```python
from build123d import *

# Parameters (mm, degrees)
F0_W      = 85
F0_H      = 117
F1_DEPTH  = 4
F2_W      = 2
F2_H      = 5
F3_DEPTH  = 7
F4_W      = 2
F4_H      = 4.0044696238
F5_DEPTH  = 5
F6_R      = 1
F7_R      = 1
F8_R      = 2
F11_W     = 117
F11_H     = 4
F12_DEPTH = 3
F10_W     = 117
F10_H     = 4
F14_DEPTH = 3
F13_W     = 85
F13_H     = 3
F13_W_2   = 3
F13_H_2   = 117
F15_DEPTH = 25
F16_DEPTH = 3
F18_DEPTH = 3
F19_R     = 0.75
F20_DEPTH = 4
F21_DEPTH = 3
F23_DEPTH = 3


# Not quite as in the source:
# - a feature names something its author has since deleted; it is built from what else it names


with BuildPart() as f1:
    # F0 (on Top) → F1 (new body)
    with BuildSketch(Plane.XY):
        Rectangle(F0_W, F0_H)
    extrude(amount=F1_DEPTH)

    # F2 (on face) → F3 (join)
    with BuildSketch(Plane(origin=(0, 0, 0), x_dir=(1, 0, 0), z_dir=(0, 0, -1))):
        with Locations((-21, -36)):
            Rectangle(F2_W, F2_H)
    extrude(amount=F3_DEPTH)

    # F4 (on face) → F5 (join)
    with BuildSketch(Plane(origin=(0, 38.5, 0), x_dir=(-1, 0, 0), z_dir=(0, 1, 0))):
        with Locations((21, -4.9977651881)):
            Rectangle(F4_W, F4_H)
    extrude(amount=F5_DEPTH)

    # F6
    f6_edges = [f1.edges().sort_by_distance(p)[0] for p in [
        (-21, 43.5, -2.99553),
    ]]
    fillet(f6_edges, radius=F6_R)

    # F7
    f7_edges = [f1.edges().sort_by_distance(p)[0] for p in [
        (-21, 43.5, -7),
    ]]
    fillet(f7_edges, radius=F7_R)

    # F8
    f8_edges = [f1.edges().sort_by_distance(p)[0] for p in [
        (-21, 33.5, -7),
    ]]
    fillet(f8_edges, radius=F8_R)


with BuildPart() as f9_1:
    # F9: instance of F1
    add(f1.part.mirror(Plane.YZ))


with BuildPart() as f1_1:
    add(f1.part)

    add(f9_1.part)  # F12 merges F9_1
    # F11 (on face) → F12 (join)
    with BuildSketch(Plane(origin=(-42.5, 0, 0), x_dir=(0, -1, 0), z_dir=(-1, 0, 0))):
        with Locations((0, 2)):
            Rectangle(F11_W, F11_H)
    extrude(amount=F12_DEPTH)

    # F10 (on face) → F14 (join)
    with BuildSketch(Plane.YZ.offset(42.5)):
        with Locations((0, 2)):
            Rectangle(F10_W, F10_H)
    extrude(amount=F14_DEPTH)

    # F13 (on face) → F15 (join)
    with BuildSketch(Plane(origin=(0, 0, 0), x_dir=(1, 0, 0), z_dir=(0, 0, -1))):
        with Locations((0, 60)):
            Rectangle(F13_W, F13_H)
        with Locations((0, -60)):
            Rectangle(F13_W, F13_H)
        with Locations((-44, 0)):
            Rectangle(F13_W_2, F13_H_2)
        with Locations((44, 0)):
            Rectangle(F13_W_2, F13_H_2)
    extrude(amount=F15_DEPTH)

    # F16 (add): a face of the model
    f16_faces = [f1_1.faces().sort_by_distance(p)[0] for p in [
        (0, 58.5, 0.9550916186),
    ]]
    extrude(f16_faces, amount=F16_DEPTH)

    # F17 (on face) → F18 (cut)
    with BuildSketch(Plane(origin=(0, 61.5, 0), x_dir=(-1, 0, 0), z_dir=(0, 1, 0))):
        Polygon((-29.3773965985, -11.6825154486), (-42.3773965985, -11.6825154486), (-42.3773965985, -17.6825154486), (-37.6342944801, -17.6825154486), (-37.6342944801, -20.6825154486), (-34.6342944801, -20.6825154486), (-34.6342944801, -17.6825154486), (-29.3773965985, -17.6825154486), align=None)
    extrude(amount=-F18_DEPTH, mode=Mode.SUBTRACT)

    # F19 (on face) → F20 (cut, through all)
    with BuildSketch(Plane.XY.offset(4)):
        with Locations((30.7380352169, -49.2682121694)):
            Circle(F19_R)
    extrude(amount=-F20_DEPTH, mode=Mode.SUBTRACT)

    # F21 (add): a face of the model
    f21_faces = [f1_1.faces().sort_by_distance(p)[0] for p in [
        (-44.5449083814, -58.5, -10.5),
    ]]
    extrude(f21_faces, amount=F21_DEPTH)

    # F22 (on face) → F23 (cut, through all)
    with BuildSketch(Plane.XZ.offset(61.5)):
        with BuildLine():
            Line((40.9117795325, -25), (40.9117795325, -9.155403553))
            ThreePointArc((40.9117795325, -9.155403553), (35.4678711158, -3.59895141), (30.1197935699, -9.2477004601))
            Line((30.1197935699, -9.2477004601), (30.1197935699, -25))
            Line((30.1197935699, -25), (40.9117795325, -25))
        make_face()
    extrude(amount=-F23_DEPTH, mode=Mode.SUBTRACT)


solid = f1_1.part
```
Geometry check sheet. Reference: the model listing, model coordinates, mm. A direction names the side the tool comes from. Coordinates: 2 decimals unless noted, no trailing zeros. Order: outer loops, then holes, each group sorted by start corner. A loop starts at its lowest first (then second) coordinate and runs counter-clockwise, first axis right, second up. Notation, with made-up numbers: (59, -24.75) - (109, -24.75) arc R21 ccw to (109, -13.75) - close; hole circle Ø5 at (59.5, -14). An arc over 180 degrees is marked (long way). Answer in a Markdown table with one row per item. Add a question column.
1. Gauge pin test, flat ends, axial feed: pin 1 Ø0.6 at (x, y) = (-21, 39.5) entering from -Z; pin 2 Ø1.2 at (x, y) = (30.74, -49.27) entering from -Z; pin 3 Ø5 at (x, y) = (13.5, 21.5) entering from -Z. Record the tip position at first contact, or that the pin passes through.
2. Draft check along Y on faces 4 (the face through (36, 60, -20.683)), 5 (the face through (-1, 61.5, -10)), 6 (the face through (-42.5, 1, -12)). Enter one of: +Y half, -Y half, draft (parallel to the pull), parting line (faces both ways), or undercut.
3. Section check B-B (x = 7). Enter the section's corners in (y, z).
4. Access from +Z, -Z, +X, -X, +Y, -Y to the whole of each face (thin tool, end or side, straight path). Record for faces 1 (the face through (37.634, 60, -19)), 2 (the face through (36, 60, -11.683)), 3 (the face through (-1, -58.5, -12)).
5. Material ranges on L1, parallel to X at y = -3.5, z = -11; L2, parallel to X at y = 35.5, z = -1.5; L3, parallel to Y at x = -41.5, z = -7.25, recorded low to high. Write a range as [from, to].
6. Section check C-C (y = -39.5). Enter the section's corners in (x, z).
7. Section check A-A (z = -15.25). Enter the section's corners in (x, y), plus the area to 3 significant figures.
Data:
| question | item | result |
|---|---|---|
| 1 | pin 1 | stops at z = -7 |
| 1 | pin 2 | passes through |
| 1 | pin 3 | stops at z = 0 |
| 2 | face 4 | draft |
| 2 | face 5 | +Y half |
| 2 | face 6 | undercut |
| 3 | outline | (-61.5, -25) - (-58.5, -25) - (-58.5, 0) - (58.5, 0) - (58.5, -25) - (61.5, -25) - (61.5, 4) - (-61.5, 4) - close |
| 4 | face 1 | +Y, -Y |
| 4 | face 2 | +Y |
| 4 | face 3 | -Z |
| 5 | L1 | x = [-45.5, -42.5], [42.5, 45.5] |
| 5 | L2 | x = [-45.5, -42.5], [-22, -20], [20, 22], [42.5, 45.5] |
| 5 | L3 | y = [-61.5, -58.5], [58.5, 61.5] |
| 6 | outline | (-45.5, -25) - (-42.5, -25) - (-42.5, 0) - (42.5, 0) - (42.5, -25) - (45.5, -25) - (45.5, 4) - (-45.5, 4) - close |
| 7 | outline | (-45.5, -61.5) - (30.12, -61.5) - (30.12, -58.5) - (-42.5, -58.5) - (-42.5, 58.5) - (29.38, 58.5) - (29.38, 61.5) - (-45.5, 61.5) - close; (40.91, -61.5) - (45.5, -61.5) - (45.5, 61.5) - (42.38, 61.5) - (42.38, 58.5) - (42.5, 58.5) - (42.5, -58.5) - (40.91, -58.5) - close |
| 7 | area | 1,180 mm² |
